```python
from build123d import *

# Parameters (mm, degrees)
EXTRUDE1_DEPTH     = 220
LPATTERN1_COUNT    = 4
LPATTERN1_PITCH    = 60
SKETCH3_R          = 82.349198064
CUT_EXTRUDE1_DEPTH = 118.39956


with BuildPart() as part:
    # Sketch1 → Extrude1 (new body)
    with BuildSketch(Plane(origin=(-20, 0, 0), x_dir=(1, 0, 0), z_dir=(0, 0, 1))):
        with BuildLine():
            Line((10, 4.000077248), (10, 1))
            Line((10, 1), (11, 0))
            Line((11, 0), (17, 0))
            Line((17, 0), (17.5, 0.5))
            Line((17.5, 0.5), (22.5, 0.5))
            Line((22.5, 0.5), (23, 0))
            Line((23, 0), (29, 0))
            Line((29, 0), (30, 1))
            Line((30, 1), (30, 4.000077248))
            Line((30, 4.000077248), (26.550048828, 7.449951172))
            Line((26.550048828, 7.449951172), (26.550048828, 10.379235268))
            Line((26.550048828, 10.379235268), (27.767930373, 11.595131504))
            ThreePointArc((27.767930373, 11.595131504), (28.341068744, 12.731631743), (29.472673258, 13.314376637))
            Line((29.472673258, 13.314376637), (30, 13.82918644))
            Line((30, 13.82918644), (30, 15.160037041))
            Line((30, 15.160037041), (29.472673258, 15.687363783))
            ThreePointArc((29.472673258, 15.687363783), (28.344874488, 16.264307267), (27.767930373, 17.392105714))
            Line((27.767930373, 17.392105714), (27.160036564, 18))
            Line((27.160036564, 18), (12.839963436, 18))
            Line((12.839963436, 18), (12.232069627, 17.392105714))
            ThreePointArc((12.232069627, 17.392105714), (11.655125512, 16.264307267), (10.527326742, 15.687363783))
            Line((10.527326742, 15.687363783), (10, 15.160037041))
            Line((10, 15.160037041), (10, 13.82918644))
            Line((10, 13.82918644), (10.527326742, 13.314376637))
            ThreePointArc((10.527326742, 13.314376637), (11.658931256, 12.731631743), (12.232069627, 11.595131504))
            Line((12.232069627, 11.595131504), (13.449951172, 10.379235268))
            Line((13.449951172, 10.379235268), (13.449951172, 7.449951172))
            Line((13.449951172, 7.449951172), (10, 4.000077248))
        make_face()
    extrude(amount=-EXTRUDE1_DEPTH)

    # Sketch2 → Cut-Revolve1 (revolve, cut)
    with BuildSketch(Plane(origin=(0, 0, 0), x_dir=(0, 0, -1), z_dir=(1, 0, 0)), mode=Mode.PRIVATE) as cut_revolve1_sk:
        Polygon((20, 18), (24.75, 18), (24.75, 9.5), (23, 9.5), (23, 0), (20, 0), align=None)
    cut_revolve1 = revolve(cut_revolve1_sk.sketch.rotate(Axis((0, 0, -20), (0, 1, 0)), 180), axis=Axis((0, 0, -20), (0, 1, 0)), mode=Mode.SUBTRACT)

    # LPattern1: Cut-Revolve1 ×4
    with Locations(*[(0, 0, -i * LPATTERN1_PITCH) for i in range(1, LPATTERN1_COUNT)]):
        add(cut_revolve1, mode=Mode.SUBTRACT)

    # Sketch3 → Cut-Extrude1 (cut)
    with BuildSketch(Plane(origin=(7.767930373, 17.392105714, 0), x_dir=(1, 0, 0), z_dir=(0, 0, 1))):
        with Locations((-44.089026553, 19.698119616)):
            Circle(SKETCH3_R)
    extrude(amount=-CUT_EXTRUDE1_DEPTH, mode=Mode.SUBTRACT)


solid = part.part
```
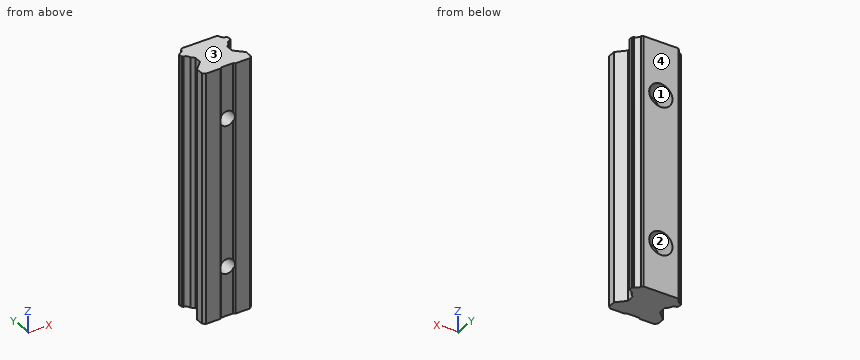
Geometry check sheet. Reference: the model listing, model coordinates, mm. Face numbers are marked on the shaded views. Coordinates: 2 decimals unless noted, no trailing zeros. Order: outer loops, then holes, each group sorted by start corner. A loop starts at its lowest first (then second) coordinate and runs counter-clockwise, first axis right, second up. Notation, with made-up numbers: (73, -1) - (124, -1) arc R27 ccw to (124, 31) - close; hole circle Ø10 at (79.25, -27). An arc over 180 degrees is marked (long way). Use one line per item in the form item = value.
1. Gauge pin test, flat ends, axial feed: pin 1 (3 mm diameter, centred on y = 8, z = -139.5, fed in from -X); pin 2 (6 mm diameter, centred on y = 8, z = -188.5, fed in from -X); pin 3 (7.5 mm diameter, centred on x = 0, z = -200, fed in from -Y); pin 4 (3 mm diameter, centred on x = 2, z = -139.5, fed in from +Y). Record the tip position at first contact, or that the pin passes through.
Here are the results:
pin_1 = -7.5
pin_2 = -9
pin_3 = 0
pin_4 = 9.5
2. Scan lines: line 1 (Z direction, x = 0, y = 4.5); line 2 (Z direction, x = -2.5, y = 6.25); line 3 (X direction, y = 3.5, z = -140). Record each from-to range of solid material in increasing order.
Here are the results:
line_1 = -220 to -203, -197 to -143, -137 to -118.4
line_2 = -220 to -201.66, -198.34 to -141.66, -138.34 to -118.4
line_3 = -10 to -3, 3 to 10
3. Section check B-B (z = -212.5). Record the boundary of the cut face in (x, y), then the cut area to 3 significant figures.
Here are the results:
outline = (-10, 1) - (-9, 0) - (-3, 0) - (-2.5, 0.5) - (2.5, 0.5) - (3, 0) - (9, 0) - (10, 1) - (10, 4) - (6.55, 7.45) - (6.55, 10.38) - (7.77, 11.6) arc R2.06 cw to (9.47, 13.31) - (10, 13.83) - (10, 15.16) - (9.47, 15.69) arc R2.06 cw to (7.77, 17.39) - (7.16, 18) - (-7.16, 18) - (-7.77, 17.39) arc R2.06 cw to (-9.47, 15.69) - (-10, 15.16) - (-10, 13.83) - (-9.47, 13.31) arc R2.06 cw to (-7.77, 11.6) - (-6.55, 10.38) - (-6.55, 7.45) - (-10, 4) - close
area = 302 mm²
4. Section check A-A (x = 0). Record the boundary of the cut face in (y, z), then the cut area to 3 significant figures.
Here are the results:
outline = (0.5, -220) - (18, -220) - (18, -204.75) - (9.5, -204.75) - (9.5, -203) - (0.5, -203) - close; (0.5, -197) - (9.5, -197) - (9.5, -195.25) - (18, -195.25) - (18, -144.75) - (9.5, -144.75) - (9.5, -143) - (0.5, -143) - close; (0.5, -137) - (9.5, -137) - (9.5, -135.25) - (18, -135.25) - (18, -118.4) - (0.5, -118.4) - close
area = 1,510 mm²
5. Draft check along Z on the marked faces 1, 2, 3 and 4. Enter one of: pulls with the +Z half, pulls with the -Z half, needs draft (parallel to the pull), parting line crosses it, or undercut.
Here are the results:
face_1 = undercut
face_2 = undercut
face_3 = pulls with the +Z half
face_4 = needs draft
